Can you work these out from the model? Positions are in its coordinate system, mm. A direction names the side the tool comes from. Give positions to 0.01 mm unless a question says otherwise; leave off trailing zeros. Write each loop counter-clockwise with the first axis right and the second up, starting at its lowest first coordinate (ties: lowest second). Pieces come first, ordered by that corner, then holes. Notation, with made-up numbers: M -3,77.25 L 32,77.25 A13 ccw 32,91.25 Z; hole C 53,71.25 d3. An arc over 180 degrees is marked long. Use CSV: the item, a comma, the result in double quotes. Start each with the question number.
from build123d import *

# Parameters (mm, degrees)
SKETCH1_W           = 36
SKETCH1_H           = 20
BOSS_EXTRUDE1_DEPTH = 15
SKETCH2_W           = 23.5
SKETCH2_H           = 20
CUT_EXTRUDE1_DEPTH  = 13
SKETCH3_R           = 1.65
CUT_EXTRUDE2_DEPTH  = 44.829214002
SKETCH4_W           = 20
SKETCH4_H           = 12
CUT_EXTRUDE3_DEPTH  = 44.829214002
SKETCH5_W           = 10
SKETCH5_H           = 20
BOSS_EXTRUDE2_DEPTH = 8
SKETCH6_R           = 1.6
CUT_EXTRUDE4_DEPTH  = 48.16990566
SKETCH7_W           = 16
SKETCH7_H           = 4
BOSS_EXTRUDE3_DEPTH = 6
FILLET1_R           = 4
FILLET2_R           = 4
FILLET5_R           = 4
SKETCH8_W           = 5.8
SKETCH8_H           = 5
BOSS_EXTRUDE4_DEPTH = 36
SKETCH9_W           = 23.5
SKETCH9_H           = 1.8
CUT_EXTRUDE5_DEPTH  = 48.091825193


# Some blends are built 0.0001 mm under size
with BuildPart() as part:
    # Sketch1 → Boss-Extrude1 (new body)
    with BuildSketch(Plane(origin=(0, 0, 0), x_dir=(1, 0, 0), z_dir=(0, 1, 0))):
        with Locations((18, -10)):
            Rectangle(SKETCH1_W, SKETCH1_H)
    extrude(amount=BOSS_EXTRUDE1_DEPTH)

    # Sketch2 → Cut-Extrude1 (cut)
    with BuildSketch(Plane(origin=(0, 0, 0), x_dir=(-1, 0, 0), z_dir=(0, -1, 0))):
        with Locations((-18, -10)):
            Rectangle(SKETCH2_W, SKETCH2_H)
    extrude(amount=-CUT_EXTRUDE1_DEPTH, mode=Mode.SUBTRACT)

    # Sketch3 → Cut-Extrude2 (cut, through all)
    with BuildSketch(Plane.ZY):
        with Locations((10, 6)):
            Circle(SKETCH3_R)
    extrude(amount=-CUT_EXTRUDE2_DEPTH, mode=Mode.SUBTRACT)

    # Sketch4 → Cut-Extrude3 (cut, through all)
    with BuildSketch(Plane(origin=(0, 15, 0), x_dir=(1, 0, 0), z_dir=(0, 1, 0))):
        with Locations((18, -10)):
            Rectangle(SKETCH4_W, SKETCH4_H)
    extrude(amount=-CUT_EXTRUDE3_DEPTH, mode=Mode.SUBTRACT)

    # Sketch5 → Boss-Extrude2 (add)
    with BuildSketch(Plane(origin=(0, 15, 0), x_dir=(1, 0, 0), z_dir=(0, 1, 0))):
        with Locations((31, -10)):
            Rectangle(SKETCH5_W, SKETCH5_H)
        with Locations((5, -10)):
            Rectangle(SKETCH5_W, SKETCH5_H)
    extrude(amount=BOSS_EXTRUDE2_DEPTH)

    # Sketch6 → Cut-Extrude4 (cut, through all)
    with BuildSketch(Plane(origin=(0, 0, 0), x_dir=(-1, 0, 0), z_dir=(0, 0, -1))):
        with Locations((-29, 18)):
            Circle(SKETCH6_R)
        with Locations((-7, 18)):
            Circle(SKETCH6_R)
    extrude(amount=-CUT_EXTRUDE4_DEPTH, mode=Mode.SUBTRACT)

    # Sketch7 → Boss-Extrude3 (add)
    with BuildSketch(Plane(origin=(0, 15, 0), x_dir=(1, 0, 0), z_dir=(0, 1, 0))):
        with Locations((18, -18)):
            Rectangle(SKETCH7_W, SKETCH7_H)
        with Locations((18, -2)):
            Rectangle(SKETCH7_W, SKETCH7_H)
    extrude(amount=BOSS_EXTRUDE3_DEPTH)

    # Fillet1
    # the kernel refuses this fillet: 4 mm, written as the material it takes off along each edge
    with BuildSketch(Plane(origin=(8, 13, 16), x_dir=(0, 0, 1), z_dir=(1, 0, 0))) as fillet1_piece_1_section:
        with BuildLine():
            CenterArc((FILLET1_R, -FILLET1_R), FILLET1_R, 90, 90)
            Line((0, -FILLET1_R), (0, 0))
            Line((0, 0), (FILLET1_R, 0))
        make_face()
    fillet1_piece_1 = extrude(amount=20, mode=Mode.PRIVATE)
    fillet1_piece_1 = split(fillet1_piece_1, bisect_by=Plane(origin=(10, 13, 16), z_dir=(-1, 0, 0)), keep=Keep.TOP, mode=Mode.PRIVATE)
    fillet1_piece_1 = split(fillet1_piece_1, bisect_by=Plane(origin=(8, 15, 16), z_dir=(0, -1, 0)), keep=Keep.TOP, mode=Mode.PRIVATE)
    add(fillet1_piece_1, mode=Mode.SUBTRACT)
    with BuildSketch(Plane(origin=(8, 13, 16), x_dir=(0, 0, 1), z_dir=(1, 0, 0))) as fillet1_piece_2_section:
        with BuildLine():
            CenterArc((FILLET1_R, -FILLET1_R), FILLET1_R, 90, 90)
            Line((0, -FILLET1_R), (0, 0))
            Line((0, 0), (FILLET1_R, 0))
        make_face()
    fillet1_piece_2 = extrude(amount=20, mode=Mode.PRIVATE)
    fillet1_piece_2 = split(fillet1_piece_2, bisect_by=Plane(origin=(10, 13, 16), z_dir=(1, 0, 0)), keep=Keep.TOP, mode=Mode.PRIVATE)
    fillet1_piece_2 = split(fillet1_piece_2, bisect_by=Plane(origin=(26, 13, 16), z_dir=(-1, 0, 0)), keep=Keep.TOP, mode=Mode.PRIVATE)
    fillet1_piece_2 = split(fillet1_piece_2, bisect_by=Plane(origin=(8, 15, 16), z_dir=(0, -1, 0)), keep=Keep.TOP, mode=Mode.PRIVATE)
    add(fillet1_piece_2, mode=Mode.SUBTRACT)
    with BuildSketch(Plane(origin=(8, 13, 16), x_dir=(0, 0, 1), z_dir=(1, 0, 0))) as fillet1_piece_3_section:
        with BuildLine():
            CenterArc((FILLET1_R, -FILLET1_R), FILLET1_R, 90, 90)
            Line((0, -FILLET1_R), (0, 0))
            Line((0, 0), (FILLET1_R, 0))
        make_face()
    fillet1_piece_3 = extrude(amount=20, mode=Mode.PRIVATE)
    fillet1_piece_3 = split(fillet1_piece_3, bisect_by=Plane(origin=(10, 13, 16), z_dir=(1, 0, 0)), keep=Keep.TOP, mode=Mode.PRIVATE)
    fillet1_piece_3 = split(fillet1_piece_3, bisect_by=Plane(origin=(26, 13, 16), z_dir=(-1, 0, 0)), keep=Keep.TOP, mode=Mode.PRIVATE)
    fillet1_piece_3 = split(fillet1_piece_3, bisect_by=Plane(origin=(8, 15, 16), z_dir=(0, 1, 0)), keep=Keep.TOP, mode=Mode.PRIVATE)
    add(fillet1_piece_3, mode=Mode.SUBTRACT)
    with BuildSketch(Plane(origin=(8, 13, 16), x_dir=(0, 0, 1), z_dir=(1, 0, 0))) as fillet1_piece_4_section:
        with BuildLine():
            CenterArc((FILLET1_R, -FILLET1_R), FILLET1_R, 90, 90)
            Line((0, -FILLET1_R), (0, 0))
            Line((0, 0), (FILLET1_R, 0))
        make_face()
    fillet1_piece_4 = extrude(amount=20, mode=Mode.PRIVATE)
    fillet1_piece_4 = split(fillet1_piece_4, bisect_by=Plane(origin=(26, 13, 16), z_dir=(1, 0, 0)), keep=Keep.TOP, mode=Mode.PRIVATE)
    fillet1_piece_4 = split(fillet1_piece_4, bisect_by=Plane(origin=(8, 15, 16), z_dir=(0, -1, 0)), keep=Keep.TOP, mode=Mode.PRIVATE)
    add(fillet1_piece_4, mode=Mode.SUBTRACT)
    with BuildSketch(Plane(origin=(28, 13, 4), x_dir=(0, 0, -1), z_dir=(-1, 0, 0))) as fillet1_piece_5_section:
        with BuildLine():
            CenterArc((FILLET1_R, -FILLET1_R), FILLET1_R, 90, 90)
            Line((0, -FILLET1_R), (0, 0))
            Line((0, 0), (FILLET1_R, 0))
        make_face()
    fillet1_piece_5 = extrude(amount=20, mode=Mode.PRIVATE)
    fillet1_piece_5 = split(fillet1_piece_5, bisect_by=Plane(origin=(26, 13, 4), z_dir=(1, 0, 0)), keep=Keep.TOP, mode=Mode.PRIVATE)
    fillet1_piece_5 = split(fillet1_piece_5, bisect_by=Plane(origin=(28, 15, 4), z_dir=(0, -1, 0)), keep=Keep.TOP, mode=Mode.PRIVATE)
    add(fillet1_piece_5, mode=Mode.SUBTRACT)
    with BuildSketch(Plane(origin=(28, 13, 4), x_dir=(0, 0, -1), z_dir=(-1, 0, 0))) as fillet1_piece_6_section:
        with BuildLine():
            CenterArc((FILLET1_R, -FILLET1_R), FILLET1_R, 90, 90)
            Line((0, -FILLET1_R), (0, 0))
            Line((0, 0), (FILLET1_R, 0))
        make_face()
    fillet1_piece_6 = extrude(amount=20, mode=Mode.PRIVATE)
    fillet1_piece_6 = split(fillet1_piece_6, bisect_by=Plane(origin=(10, 13, 4), z_dir=(1, 0, 0)), keep=Keep.TOP, mode=Mode.PRIVATE)
    fillet1_piece_6 = split(fillet1_piece_6, bisect_by=Plane(origin=(26, 13, 4), z_dir=(-1, 0, 0)), keep=Keep.TOP, mode=Mode.PRIVATE)
    fillet1_piece_6 = split(fillet1_piece_6, bisect_by=Plane(origin=(28, 15, 4), z_dir=(0, -1, 0)), keep=Keep.TOP, mode=Mode.PRIVATE)
    add(fillet1_piece_6, mode=Mode.SUBTRACT)
    with BuildSketch(Plane(origin=(28, 13, 4), x_dir=(0, 0, -1), z_dir=(-1, 0, 0))) as fillet1_piece_7_section:
        with BuildLine():
            CenterArc((FILLET1_R, -FILLET1_R), FILLET1_R, 90, 90)
            Line((0, -FILLET1_R), (0, 0))
            Line((0, 0), (FILLET1_R, 0))
        make_face()
    fillet1_piece_7 = extrude(amount=20, mode=Mode.PRIVATE)
    fillet1_piece_7 = split(fillet1_piece_7, bisect_by=Plane(origin=(10, 13, 4), z_dir=(1, 0, 0)), keep=Keep.TOP, mode=Mode.PRIVATE)
    fillet1_piece_7 = split(fillet1_piece_7, bisect_by=Plane(origin=(26, 13, 4), z_dir=(-1, 0, 0)), keep=Keep.TOP, mode=Mode.PRIVATE)
    fillet1_piece_7 = split(fillet1_piece_7, bisect_by=Plane(origin=(28, 15, 4), z_dir=(0, 1, 0)), keep=Keep.TOP, mode=Mode.PRIVATE)
    add(fillet1_piece_7, mode=Mode.SUBTRACT)
    with BuildSketch(Plane(origin=(28, 13, 4), x_dir=(0, 0, -1), z_dir=(-1, 0, 0))) as fillet1_piece_8_section:
        with BuildLine():
            CenterArc((FILLET1_R, -FILLET1_R), FILLET1_R, 90, 90)
            Line((0, -FILLET1_R), (0, 0))
            Line((0, 0), (FILLET1_R, 0))
        make_face()
    fillet1_piece_8 = extrude(amount=20, mode=Mode.PRIVATE)
    fillet1_piece_8 = split(fillet1_piece_8, bisect_by=Plane(origin=(10, 13, 4), z_dir=(-1, 0, 0)), keep=Keep.TOP, mode=Mode.PRIVATE)
    fillet1_piece_8 = split(fillet1_piece_8, bisect_by=Plane(origin=(28, 15, 4), z_dir=(0, -1, 0)), keep=Keep.TOP, mode=Mode.PRIVATE)
    add(fillet1_piece_8, mode=Mode.SUBTRACT)

    # Fillet2
    # the kernel refuses this fillet: 4 mm, written as the material it adds along each edge
    with BuildSketch(Plane(origin=(8, 15, 21.535898385), x_dir=(1, 0, 0), z_dir=(0, 0, -1))) as fillet2_piece_1_section:
        with BuildLine():
            CenterArc((3.645751311, 3.645751311), FILLET2_R, 204.295188945, 41.409622109)
            Line((0, 2), (0, 0))
            Line((0, 0), (2, 0))
        make_face()
    fillet2_piece_1 = extrude(amount=23.07179677, mode=Mode.PRIVATE)
    fillet2_piece_1 = split(fillet2_piece_1, bisect_by=Plane(origin=(8, 15, 0), z_dir=(0, 0, 1)), keep=Keep.TOP, mode=Mode.PRIVATE)
    fillet2_piece_1 = split(fillet2_piece_1, bisect_by=Plane(origin=(8, 15, 20), z_dir=(0, 0, -1)), keep=Keep.TOP, mode=Mode.PRIVATE)
    add(fillet2_piece_1)
    with BuildSketch(Plane(origin=(28, 15, -1.535898385), x_dir=(-1, 0, 0), z_dir=(0, 0, 1))) as fillet2_piece_2_section:
        with BuildLine():
            CenterArc((3.645751311, 3.645751311), FILLET2_R, 204.295188945, 41.409622109)
            Line((0, 2), (0, 0))
            Line((0, 0), (2, 0))
        make_face()
    fillet2_piece_2 = extrude(amount=23.07179677, mode=Mode.PRIVATE)
    fillet2_piece_2 = split(fillet2_piece_2, bisect_by=Plane(origin=(28, 15, 0), z_dir=(0, 0, 1)), keep=Keep.TOP, mode=Mode.PRIVATE)
    fillet2_piece_2 = split(fillet2_piece_2, bisect_by=Plane(origin=(28, 15, 20), z_dir=(0, 0, -1)), keep=Keep.TOP, mode=Mode.PRIVATE)
    add(fillet2_piece_2)

    # Fillet5
    fillet5_edges = [part.edges().sort_by_distance(p)[0] for p in [
        (18, 21, 16),
        (18, 21, 4),
    ]]
    fillet(fillet5_edges, radius=FILLET5_R - 0.0001)  # a hair under: the kernel refuses the full size

    # Sketch8 → Boss-Extrude4 (add)
    with BuildSketch(Plane.ZY):
        with Locations((22.9, 9.5)):
            Rectangle(SKETCH8_W, SKETCH8_H)
        with Locations((-2.9, 9.5)):
            Rectangle(SKETCH8_W, SKETCH8_H)
    extrude(amount=-BOSS_EXTRUDE4_DEPTH)

    # Sketch9 → Cut-Extrude5 (cut, through all)
    with BuildSketch(Plane(origin=(0, 7, 0), x_dir=(-1, 0, 0), z_dir=(0, -1, 0))):
        with Locations((-18, 0.9)):
            Rectangle(SKETCH9_W, SKETCH9_H)
        with Locations((-18, -20.9)):
            Rectangle(SKETCH9_W, SKETCH9_H)
    extrude(amount=-CUT_EXTRUDE5_DEPTH, mode=Mode.SUBTRACT)


solid = part.part
(1) I want a section at A-A (z = 10). Write out the boundary of the cut face in (x, y), and give its area (3 significant figures).
(2) Which directions (+Z, -Z, +X, -X, +Y, -Y) give clear straight access to the entire face, cutting with the end or side of a thin tool? Please do faces 1 (the face through (18, 9, 21.8)), 2 (the face through (18.112, 19.859, 2.797)), 3 (the face through (18, 12, -4)).
(3) Thinking about a two-plate mould opening in Z: for faces 4 (the face through (3.081, 4.536, 10.761)), 5 (the face through (17.86, 14.141, 17.203)), 6 (the face through (29, 13, 10)), 7 (the face through (18, 9, -5.8)), which applies, released by +Z, released by -Z, zero draft, split by the parting line, or undercut?
(4) I want a section at B-B (y = 3.75). Write out the boundary of the cut face in (x, z).
(5) I want a section at D-D (z = 6.5). Write out the boundary of the cut face in (x, y).
(6) I want a section at C-C (x = 15). State how many separate pieces and enclosed holes the cut face has, and give its area (3 significant figures).
(7) Please list where these lines run through material, in increasing order: L1, parallel to X at y = 18, z = 11.25; L2, parallel to Y at x = 29, z = 9.5; L3, parallel to X at y = 3, z = 16. Write a range as [from, to].
(8) Will these pins go through, and if not, where does the flat tip stop? pin 1 Ø2 at (x, y) = (28, 16.5) entering from -Z; pin 2 Ø10 at (x, z) = (21, 0) entering from -Y; pin 3 Ø3 at (x, z) = (20, -2.5) entering from +Y.
Geometry results:
1,outline,"M 0,0 L 6.25,0 L 6.25,4.35 L 0,4.35 Z; M 0,7.65 L 6.25,7.65 L 6.25,13 L 8,13 A4 cw 10,15 L 10,23 L 0,23 Z; M 26,15 A4 cw 28,13 L 29.75,13 L 29.75,7.65 L 36,7.65 L 36,23 L 26,23 Z; M 29.75,0 L 36,0 L 36,4.35 L 29.75,4.35 Z; hole C 7,18 d3.2; hole C 29,18 d3.2"
1,area,"300 mm2"
2,face 1,"+Y, -Y"
2,face 2,"+Y"
2,face 3,"-Z, +X, -X, +Y"
3,face 4,"undercut"
3,face 5,"undercut"
3,face 6,"zero draft"
3,face 7,"released by -Z"
4,outline,"M 0,0 L 6.25,0 L 6.25,20 L 0,20 Z; M 29.75,0 L 36,0 L 36,20 L 29.75,20 Z"
5,outline,"M 0,0 L 6.25,0 L 6.25,13 L 8,13 A4 cw 10,15 L 10,23 L 0,23 Z; M 26,15 A4 cw 28,13 L 29.75,13 L 29.75,0 L 36,0 L 36,23 L 26,23 Z; hole C 7,18 d3.2; hole C 29,18 d3.2"
6,separate pieces,"4"
6,enclosed holes,"0"
6,area,"90.3 mm2"
7,L1,"x = [0, 5.4], [8.6, 10], [26, 27.4], [30.6, 36]"
7,L2,"y = [13, 16.4], [19.6, 23]"
7,L3,"x = [0, 6.25], [29.75, 36]"
8,pin 1,"stops at z = 0"
8,pin 2,"stops at y = 7"
8,pin 3,"stops at y = 12"
